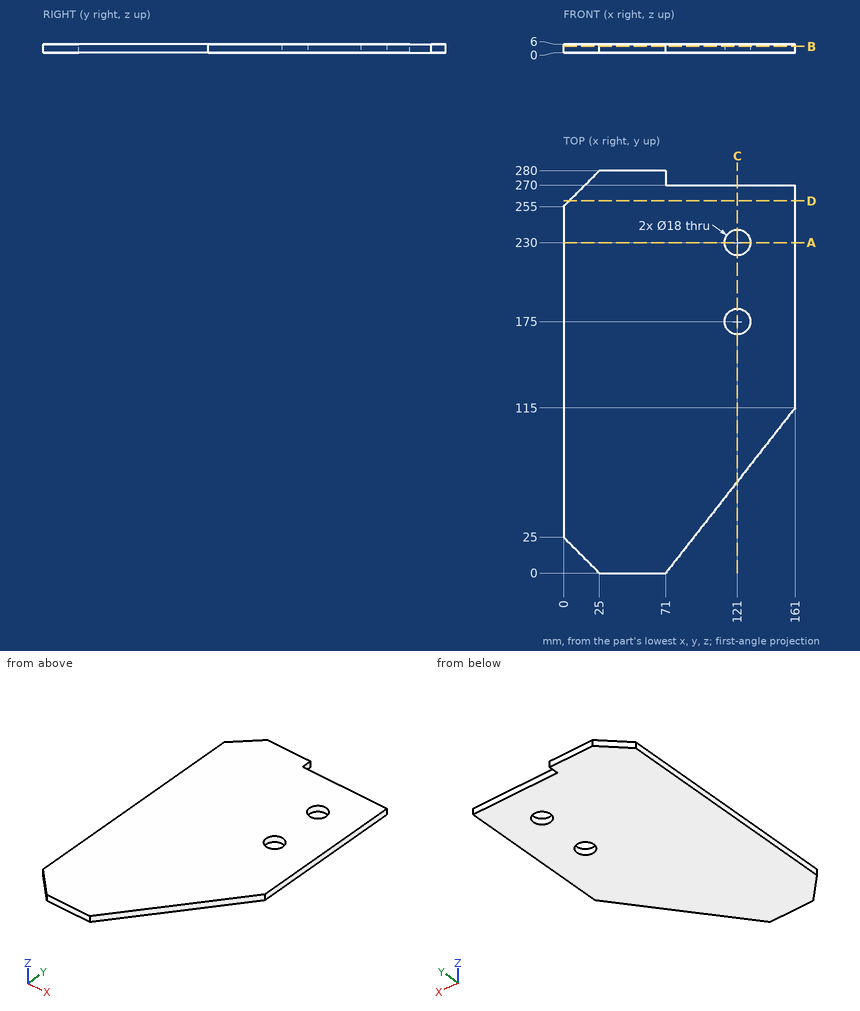
Could you check a few things on this drawing? It's one solid part, dimensions in mm from its lowest x, y, z. Coordinates: 2 decimals unless noted, no trailing zeros. Order: outer loops, then holes, each group sorted by start corner. A loop starts at its lowest first (then second) coordinate and runs counter-clockwise, first axis right, second up.
1. If we section it at C-C (x = 121): Please give me the cut outline in (y, z), then the cut area to 3 significant figures.
2. If we section it at A-A (y = 230): Please give me the cut outline in (x, z).
3. I need wall thicknesses on line 1 (Y direction, x = 121, z = 1.6); line 2 (X direction, y = 230, z = 3.7); line 3 (Y direction, x = 86, z = 4.4). Which ranges of each line are inside material? Lowest first, please.
4. If we section it at D-D (y = 259): Please give me the cut outline in (x, z).
5. If we section it at B-B (z = 4.3): Please give me the cut outline in (x, y).
6. I'm going to push flat-ended pins straight in: pin 1 (11 mm diameter, centred on x = 121, y = 175, fed in from +Z); pin 2 (1.8 mm diameter, centred on y = 276, z = 1.5, fed in from +X). Where does each tip first touch, or does it pass through?
Entries:
1. outline: (63.89, 0) - (166, 0) - (166, 6) - (63.89, 6) - close; (184, 0) - (221, 0) - (221, 6) - (184, 6) - close; (239, 0) - (270, 0) - (270, 6) - (239, 6) - close
1. area: 1,020 mm2
2. outline: (0, 0) - (112, 0) - (112, 6) - (0, 6) - close; (130, 0) - (161, 0) - (161, 6) - (130, 6) - close
3. line 1: y = 63.89 to 166, 184 to 221, 239 to 270
3. line 2: x = 0 to 112, 130 to 161
3. line 3: y = 19.17 to 270
4. outline: (4, 0) - (161, 0) - (161, 6) - (4, 6) - close
5. outline: (0, 25) - (25, 0) - (71, 0) - (161, 115) - (161, 270) - (71, 270) - (71, 280) - (25, 280) - (0, 255) - close; hole circle Ø18 at (121, 175); hole circle Ø18 at (121, 230)
6. pin 1: passes through
6. pin 2: stops at x = 71
